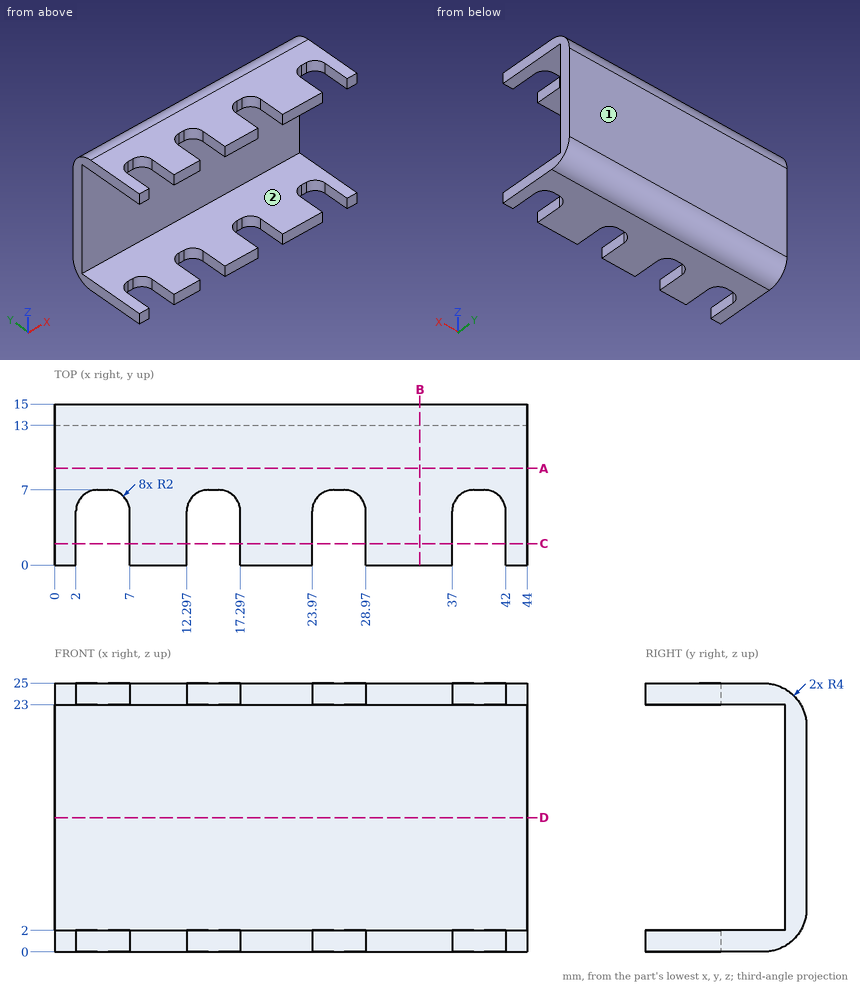
Could you check a few things on this drawing? It's one solid part, dimensions in mm from its lowest x, y, z. A direction names the side the tool comes from. Coordinates: 2 decimals unless noted, no trailing zeros. Write each loop counter-clockwise with the first axis right and the second up, starting at its lowest first coordinate (ties: lowest second). Pieces come first, ordered by that corner, then holes. Notation, with made-up numbers: (3, 17) - (15, 17) arc R15 cw to (15, 34) - close; hole circle Ø4 at (-24, 34.25). An arc over 180 degrees is marked (long way). Put each result on its own line as item: value. Start each with the question number.
Q1. I want a section at D-D on z = 12.5. Write out the boundary of the cut face in (x, y).
Q2. I want a section at A-A on y = 9. Write out the boundary of the cut face in (x, z), plus the area to 3 significant figures.
Q3. Which directions (+Z, -Z, +X, -X, +Y, -Y) give clear straight access to the entire face, cutting with the end or side of a thin tool? Please do the marked faces 1 and 2.
Q4. Please list where these lines run through material, in increasing order: L1, parallel to Z at x = 27.5, y = 8.25; L2, parallel to Y at x = 13, z = 12.75; L3, parallel to Z at x = 22.5, y = 12.25.
Q5. I want a section at C-C on y = 2. Count the separate pieces of the cut face and the enclosed holes in it.
Q6. I'm going to push flat-ended pins straight in: P1, Ø1.1, axis at x = 26.5, z = 24, coming from the -Y side; P2, Ø1.6, axis at y = 3, z = 23.5, coming from the -X side; P3, Ø3, axis at x = 11.5, z = 15, coming from the -Y side. Where does each tip first touch, or does it pass through?
Q7. I want a section at B-B on x = 34. Write out the boundary of the cut face in (y, z).
Checks:
1. outline: (0, 13) - (44, 13) - (44, 15) - (0, 15) - close
2. outline: (0, 0) - (44, 0) - (44, 2) - (0, 2) - close; (0, 23) - (44, 23) - (44, 25) - (0, 25) - close
2. area: 176 mm²
3. face 1: +Z, -Z, +X, -X, +Y
3. face 2: +X, -X, -Y
4. L1: 0 to 2, 23 to 25
4. L2: 13 to 15
4. L3: 0.2 to 2, 23 to 24.8
5. separate pieces: 10
5. enclosed holes: 0
6. P1: y = 7
6. P2: x = 0
6. P3: y = 13
7. outline: (0, 0) - (11, 0) arc R4 ccw to (15, 4) - (15, 21) arc R4 ccw to (11, 25) - (0, 25) - (0, 23) - (13, 23) - (13, 2) - (0, 2) - close
